Check sheet for the modelled part. Datum: model origin and axes. Units: mm. A direction names the side the tool comes from. Give positions to 0.01 mm unless a question says otherwise; leave off trailing zeros. Order: outer loops, then holes, each group sorted by start corner. A loop starts at its lowest first (then second) coordinate and runs counter-clockwise, first axis right, second up. Notation, with made-up numbers: (68.25, 1) -> (101.25, 1) arc R27 cw to (101.25, 40) -> close; hole circle Ø9 at (63, -39.75). An arc over 180 degrees is marked (long way). Answer in a Markdown table with one row per item. Add a question column.
(1) Cross-section at B-B (x = 0). Record the cut outline in (y, z), then the cut area to 3 significant figures.
(2) Thickness scan on L1, parallel to X at y = 1.75, z = 0; L2, parallel to Z at x = -6.5, y = 6; L3, parallel to Z at x = -13, y = 2. Record the ranges inside material, lowest first. Write a range as [from, to].
(3) Set-up check for faces 1 (the face through (-4, 6.5, 19)), 2 (the face through (19, 6.5, 4)), 3 (the face through (-7.165, 3.906, 17.821)): record each of +Z, -Z, +X, -X, +Y, -Y from which the full face is reachable in a straight line by a thin tool's end or side.
(4) Cross-section at A-A (z = 0). Record the cut outline in (x, y).
(5) Release check for a two-part mould opening along Z. For faces 4 (the face through (-6.825, 6.796, 18.045)), 5 (the face through (-13.4, 7.1, 13.9)), 6 (the face through (-13.783, 3.906, 13.5)), 7 (the face through (14, 6.8, -13.15)) record: released by +Z, released by -Z, zero draft, split by the parting line, or undercut.
(6) Cross-section at C-C (z = -12.5). Record the cut outline in (x, y), then the cut area to 3 significant figures.
(7) Go/stop test with flat-tipped pins: pin 1 (2 mm diameter, centred on x = -17, z = -3.5, fed in from +Y); pin 2 (0.7 mm diameter, centred on y = 7, z = -18.5, fed in from +X); pin 3 (0.7 mm diameter, centred on y = 7, z = 19, fed in from +X). Record where each tip stops, or that it passes through.
```python
from build123d import *
from build123d.topology import SkipClean

# Parameters (mm, degrees)
SKETCH1_R           = 22.3
SKETCH1_R_2         = 16.2
BOSS_EXTRUDE1_DEPTH = 6.5
BOSS_EXTRUDE2_DEPTH = 0.6
CIRPATTERN1_COUNT   = 16
CUT_EXTRUDE1_START  = -6.3
CUT_EXTRUDE1_DEPTH  = 6.3


with BuildPart() as part:
    # Sketch1 → Boss-Extrude1 (new body)
    with BuildSketch(Plane(origin=(0, 0, 0), x_dir=(1, 0, 0), z_dir=(0, 1, 0))):
        with Locations(Location((0, 0, 0), (0, 0, 90))):
            Circle(SKETCH1_R)
        with Locations(Location((0, 0, 0), (0, 0, 90))):
            Circle(SKETCH1_R_2, mode=Mode.SUBTRACT)
    extrude(amount=BOSS_EXTRUDE1_DEPTH)

    # Sketch2 → Boss-Extrude2 (add)
    with BuildSketch(Plane(origin=(0, 6.5, 0), x_dir=(1, 0, 0), z_dir=(0, 1, 0))):
        with BuildLine():
            ThreePointArc((0.6, 22.29192679), (0, 22.3), (-0.6, 22.29192679))
            Line((-0.6, 22.29192679), (-0.6, 16.188885076))
            ThreePointArc((-0.6, 16.188885076), (0, 16.2), (0.6, 16.188885076))
            Line((0.6, 16.188885076), (0.6, 22.29192679))
        make_face()
    boss_extrude2 = extrude(amount=BOSS_EXTRUDE2_DEPTH)

    # CirPattern1: Boss-Extrude2 ×16 about axis
    with SkipClean():  # the faces are left unmerged after this step: merging them gives an invalid solid
        cirpattern1_axis = Axis((0, 0, 0), (0, 1, 0))
        for i in range(1, CIRPATTERN1_COUNT):
            add(boss_extrude2.rotate(cirpattern1_axis, i * 360 / CIRPATTERN1_COUNT))

    # Sketch3 → Cut-Extrude1 (cut)
    with SkipClean():  # the faces are left unmerged after this step: merging them gives an invalid solid
        with BuildSketch(Plane(origin=(0, 7.1, 0), x_dir=(1, 0, 0), z_dir=(0, 1, 0)).offset(CUT_EXTRUDE1_START)):
            with BuildLine():
                Line((-15.909268387, -15.626425675), (-11.595678207, -11.312835494))
                ThreePointArc((-11.595678207, -11.312835494), (-11.455129855, -11.455129855), (-11.312835494, -11.595678207))
                Line((-11.312835494, -11.595678207), (-15.626425675, -15.909268387))
                ThreePointArc((-15.626425675, -15.909268387), (-15.76848122, -15.76848122), (-15.909268387, -15.626425675))
            make_face()
            with BuildLine():
                Line((-6.014223231, -15.042244478), (-8.348721414, -20.678221653))
                ThreePointArc((-8.348721414, -20.678221653), (-8.533840542, -20.602513575), (-8.718273228, -20.52514828))
                Line((-8.718273228, -20.52514828), (-6.383775044, -14.889171105))
                ThreePointArc((-6.383775044, -14.889171105), (-6.199471604, -14.966848427), (-6.014223231, -15.042244478))
            make_face()
        extrude(amount=CUT_EXTRUDE1_DEPTH, mode=Mode.SUBTRACT)


solid = part.part
```
Answer below:
| question | item | result |
|---|---|---|
| 1 | outline | (0, -22.3) -> (7.1, -22.3) -> (7.1, -16.2) -> (0, -16.2) -> close; (0, 16.2) -> (7.1, 16.2) -> (7.1, 22.3) -> (0, 22.3) -> close |
| 1 | area | 86.6 mm² |
| 2 | L1 | x = [-22.3, -16.2], [16.2, 22.3] |
| 2 | L2 | z = [-21.33, -14.84], [14.84, 15.17], [16.22, 21.33] |
| 2 | L3 | z = [-18.12, -9.67], [9.67, 12.72], [13.28, 18.12] |
| 3 | face 1 | +Z, +Y |
| 3 | face 2 | +X, +Y |
| 3 | face 3 | +Y |
| 4 | outline | (-22.3, 0) -> (-16.2, 0) -> (-16.2, 7.1) -> (-22.3, 7.1) -> close; (16.2, 0) -> (22.3, 0) -> (22.3, 7.1) -> (16.2, 7.1) -> close |
| 5 | face 4 | released by +Z |
| 5 | face 5 | zero draft |
| 5 | face 6 | undercut |
| 5 | face 7 | undercut |
| 6 | outline | (-18.47, 0) -> (-10.3, 0) -> (-10.3, 6.5) -> (-11.65, 6.5) -> (-11.65, 7.1) -> (-13.35, 7.1) -> (-13.35, 6.5) -> (-18.47, 6.5) -> close; (10.3, 0) -> (18.47, 0) -> (18.47, 6.5) -> (13.35, 6.5) -> (13.35, 7.1) -> (11.65, 7.1) -> (11.65, 6.5) -> (10.3, 6.5) -> close |
| 6 | area | 108 mm² |
| 7 | pin 1 | stops at y = 6.5 |
| 7 | pin 2 | stops at x = 8.46 |
| 7 | pin 3 | stops at x = 8.66 |
